Autodesk Inventor part; units mm, degrees
ref_plane "YZ Plane" through (0, 0, 0) normal (1, 0, 0) x (0, 1, 0)
ref_plane "XY Plane" through (0, 0, 0) normal (0, 0, 1) x (1, 0, 0)
sketch "Sketch1" plane through (0, 0, 0) normal (0, 1, 0) x (-1, 0, 0)
  circle A0 centre (0, 0) radius 5
  dimension "d0" = 10
extrude "Extrusion1" add sketch "Sketch1" along normal blind 35
ref_plane "Work Plane1" through (0, -5, 0) normal (0, 1, 0) x (-1, 0, 0)
sketch "Sketch4" plane through (0, -5, 0) normal (0, 1, 0) x (-1, 0, 0)
  circle A0 centre (0, 0) radius 6
  dimension "d8" = 12
loft "Loft1" add profiles "Sketch4" section 1 edges at (5, 0, 0)
ref_plane "Work Plane2" through (0, 41, 0) normal (0, 1, 0) x (1, 0, 0)
sketch "Sketch5" plane through (0, 41, 0) normal (0, 1, 0) x (1, 0, 0)
  circle A0 centre (0, 0) radius 12.5
  dimension "d14" = 25
loft "Loft2" add profiles "Sketch5" section 2 edges at (5, 35, 0)
fillet "Face Fillet1" radius 15 2 edges at (0, 35, -5) (0, 35, 5)
fillet "Face Fillet2" radius 42 1 edges at (5, 0, 0)
properties part number "table_column"
Input: part model. Units: mm. Frame: model coordinates. Coordinates: 2 decimals unless noted, no trailing zeros. Loops run counter-clockwise (first coordinate to the right, second up) from the corner with the lowest first, then second, coordinate; pieces in that order, holes last.
(1) Material intervals for probe 1 along Y at (x, z) = (-3.5, -7.25); probe 2 along Y at (x, z) = (-9.5, -2.5); probe 3 along Z at (x, y) = (-0.5, 6.5), sorted ascending.
(2) Pull-direction query (Y, two-part tool) for faces 1 (the face through (0, 41, 0)), 2 (the face through (10.25, 39.6, -3.23)), 3 (the face through (1.08, 15.81, 4.88)); classes: released by +Y, released by -Y, zero draft, split by the parting line, or undercut.
(3) First-contact query: pin 1 Ø10 at (x, y) = (8.5, 15) entering from -Z; pin 2 Ø6 at (y, z) = (20.5, 6) entering from +X; pin 3 Ø1.5 at (x, y) = (4.5, 8.5) entering from -Z. Flat tips, straight axial feed; report the tip coordinate or a pass-through.
(4) Section A-A on y = 20.5. Return the cut outline in (x, z).
Data:
1. probe 1: y = 36.86 to 41
1. probe 2: y = 38.81 to 41
1. probe 3: z = -4.97 to 4.97
2. face 1: released by +Y
2. face 2: released by -Y
2. face 3: undercut
3. pin 1: stops at z = -3.57
3. pin 2: stops at x = 4
3. pin 3: stops at z = -3.31
4. outline: circle Ø10 at (0, 0)
